The drawing under review shows one solid part. Ordinate dimensions are in mm from its lowest x, y, z. Give positions to 0.01 mm unless a question says otherwise; leave off trailing zeros. Write each loop counter-clockwise with the first axis right and the second up, starting at its lowest first coordinate (ties: lowest second). Pieces come first, ordered by that corner, then holes. Notation, with made-up numbers: (76.25, 14) -> (126.25, 14) arc R19 cw to (126.25, 47) -> close; hole circle Ø3 at (-39, 29). An arc over 180 degrees is marked (long way). Put each result on its own line as item: value. Start each with the question number.
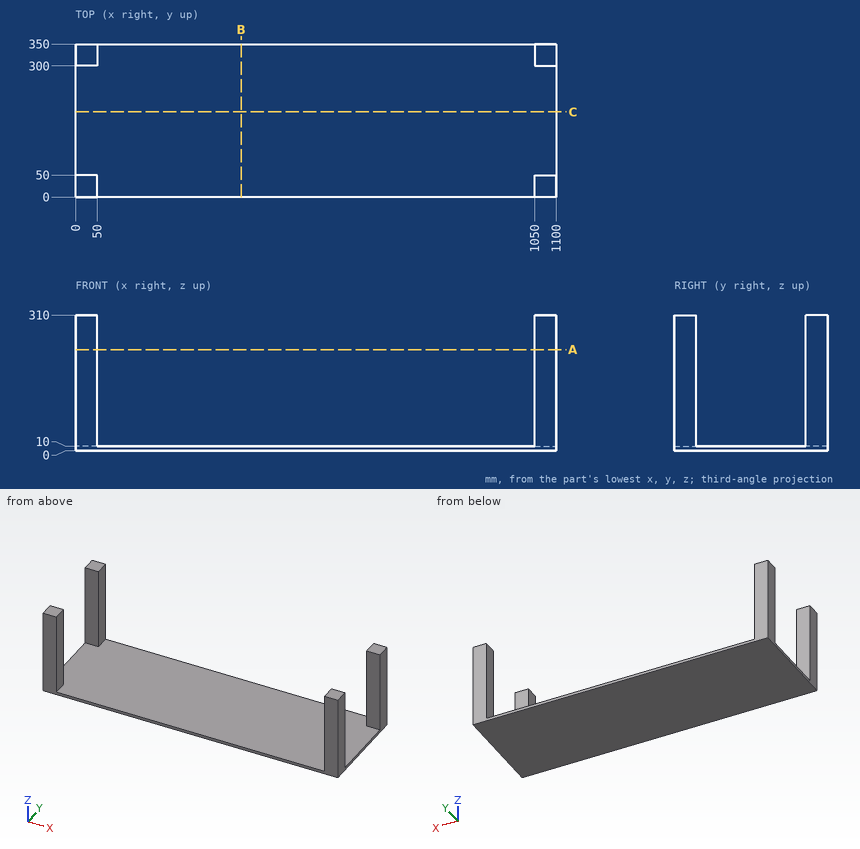
Q1. To check wall thickness, follow probe 1 along X at (y, z) = (45.5, 104); probe 2 along Z at (x, y) = (556.5, 72.5). State the ranges of each line that lie inside material, in increasing order. Write a range as from..to.
Q2. For pin 1 (2 mm diameter, centred on x = 125, y = 206.5, fed in from +Z); pin 2 (12 mm diameter, centred on x = 154, y = 154.5, fed in from -Z), all flat-tipped, find the tip position at first contact; note any pin that passes through.
Q3. Take a section at C-C on y = 195. Give the boundary of the cut face in (x, z).
Q4. Take a section at A-A on z = 231. Give the boundary of the cut face in (x, y).
Q5. Take a section at B-B on x = 379. Give the boundary of the cut face in (y, z).
Result:
1. probe 1: x = 0..50, 1050..1100
1. probe 2: z = 0..10
2. pin 1: stops at z = 10
2. pin 2: stops at z = 0
3. outline: (0, 0) -> (1100, 0) -> (1100, 10) -> (0, 10) -> close
4. outline: (0, 0) -> (50, 0) -> (50, 50) -> (0, 50) -> close; (0, 300) -> (50, 300) -> (50, 350) -> (0, 350) -> close; (1050, 0) -> (1100, 0) -> (1100, 50) -> (1050, 50) -> close; (1050, 300) -> (1100, 300) -> (1100, 350) -> (1050, 350) -> close
5. outline: (0, 0) -> (350, 0) -> (350, 10) -> (0, 10) -> close
